```python
from build123d import *

# Parameters (mm, degrees)
BOSS_EXTRUDE1_OUTLINE_W   = 188.4
BOSS_EXTRUDE1_OUTLINE_H   = 88.4
BOSS_EXTRUDE1_DEPTH       = 5.8
BOSS_EXTRUDE1_2_OUTLINE_R = 1.5
BOSS_EXTRUDE1_2_OUTLINE_W = 22.55
BOSS_EXTRUDE1_2_OUTLINE_H = 11.95
BOSS_EXTRUDE1_2_DEPTH     = 5.8
SKETCH2_W                 = 22.55
SKETCH2_H                 = 11.95
CUT_EXTRUDE1_DEPTH        = 6.35
SKETCH3_R                 = 1.5
SKETCH3_W                 = 22.55
SKETCH3_H                 = 11.95
CUT_EXTRUDE2_DEPTH        = 107.804868803
CUT_EXTRUDE3_DEPTH        = 107.804868803
SKETCH5_W                 = 5.8
SKETCH5_H                 = 188.4
BOSS_EXTRUDE2_DEPTH       = 5.8
CUT_EXTRUDE5_DEPTH        = 5.8


# Read off the part's stored shape, not the designer's step: Boss-Extrude1
with BuildPart() as part:
    # Boss-Extrude1 outline → Boss-Extrude1 (new body)
    with BuildSketch(Plane(origin=(0, 0, 0), x_dir=(0, 0, -1), z_dir=(1, 0, 0))):
        Rectangle(BOSS_EXTRUDE1_OUTLINE_W, BOSS_EXTRUDE1_OUTLINE_H)
    extrude(amount=BOSS_EXTRUDE1_DEPTH)

    # Sketch2 → Cut-Extrude1 (cut)
    with BuildSketch(Plane(origin=(5.8, 0, 0), x_dir=(0, 0, -1), z_dir=(1, 0, 0))):
        with Locations((-70.783988916, 0)):
            Rectangle(SKETCH2_W, SKETCH2_H)
    extrude(amount=-CUT_EXTRUDE1_DEPTH, mode=Mode.SUBTRACT)

    # Sketch3 → Cut-Extrude2 (cut, through all)
    with BuildSketch(Plane(origin=(5.8, 0, 0), x_dir=(0, 0, -1), z_dir=(1, 0, 0))):
        with Locations((-66.978988916, 11)):
            Circle(SKETCH3_R)
        with Locations(Location((-66.978988916, -11, 0), (0, 0, 180))):
            Circle(SKETCH3_R)
        with Locations((-70.783988916, 0)):
            Rectangle(SKETCH3_W, SKETCH3_H)
    extrude(amount=-CUT_EXTRUDE2_DEPTH, mode=Mode.SUBTRACT)

    # Sketch4 → Cut-Extrude3 (cut, through all)
    with BuildSketch(Plane(origin=(5.8, 0, 0), x_dir=(0, 0, -1), z_dir=(1, 0, 0))):
        Polygon((-94.2, 34), (-90.2, 34), (-90.2, 35.21), (-87.85, 35.21), (-87.85, 34), (-85.85, 34), (-85.85, 31), (-87.85, 31), (-87.85, 29.79), (-90.2, 29.79), (-90.2, 31), (-94.2, 31), align=None)
        Polygon((-87.85, -31), (-87.85, -29.79), (-90.2, -29.79), (-90.2, -31), (-94.2, -31), (-94.2, -34), (-90.2, -34), (-90.2, -35.21), (-87.85, -35.21), (-87.85, -34), (-85.85, -34), (-85.85, -31), align=None)
        Polygon((94.2, -34), (90.2, -34), (90.2, -35.21), (87.85, -35.21), (87.85, -34), (85.85, -34), (85.85, -31), (87.85, -31), (87.85, -29.79), (90.2, -29.79), (90.2, -31), (94.2, -31), align=None)
        Polygon((87.85, 31), (87.85, 29.79), (90.2, 29.79), (90.2, 31), (94.2, 31), (94.2, 34), (90.2, 34), (90.2, 35.21), (87.85, 35.21), (87.85, 34), (85.85, 34), (85.85, 31), align=None)
    extrude(amount=-CUT_EXTRUDE3_DEPTH, mode=Mode.SUBTRACT)



with BuildPart() as body_2:
    # Boss-Extrude1 2 outline → Boss-Extrude1 2 (new body)
    with BuildSketch(Plane(origin=(0, 0, 0), x_dir=(0, 0, -1), z_dir=(1, 0, 0))):
        Polygon((94.2, 34), (94.2, 50), (-94.2, 50), (-94.2, 34), (-90.2, 34), (-90.2, 35.21), (-87.85, 35.21), (-87.85, 34), (-85.85, 34), (-85.85, 31), (-87.85, 31), (-87.85, 29.79), (-90.2, 29.79), (-90.2, 31), (-94.2, 31), (-94.2, -31), (-90.2, -31), (-90.2, -29.79), (-87.85, -29.79), (-87.85, -31), (-85.85, -31), (-85.85, -34), (-87.85, -34), (-87.85, -35.21), (-90.2, -35.21), (-90.2, -34), (-94.2, -34), (-94.2, -44.2), (94.2, -44.2), (94.2, -34), (90.2, -34), (90.2, -35.21), (87.85, -35.21), (87.85, -34), (85.85, -34), (85.85, -31), (87.85, -31), (87.85, -29.79), (90.2, -29.79), (90.2, -31), (94.2, -31), (94.2, 31), (90.2, 31), (90.2, 29.79), (87.85, 29.79), (87.85, 31), (85.85, 31), (85.85, 34), (87.85, 34), (87.85, 35.21), (90.2, 35.21), (90.2, 34), align=None)
        with Locations((-66.978988916, -11)):
            Circle(BOSS_EXTRUDE1_2_OUTLINE_R, mode=Mode.SUBTRACT)
        with Locations((-70.783988916, 0)):
            Rectangle(BOSS_EXTRUDE1_2_OUTLINE_W, BOSS_EXTRUDE1_2_OUTLINE_H, mode=Mode.SUBTRACT)
        with Locations((-66.978988916, 11)):
            Circle(BOSS_EXTRUDE1_2_OUTLINE_R, mode=Mode.SUBTRACT)
    extrude(amount=BOSS_EXTRUDE1_2_DEPTH)


with BuildPart() as part_1:
    add(part.part)

    add(body_2.part)  # Boss-Extrude2 merges body 2
    # Sketch5 → Boss-Extrude2 (add)
    with BuildSketch(Plane(origin=(0, 44.2, 0), x_dir=(1, 0, 0), z_dir=(0, 1, 0))):
        with Locations((2.9, 0)):
            Rectangle(SKETCH5_W, SKETCH5_H)
    extrude(amount=BOSS_EXTRUDE2_DEPTH)

    # Sketch8 → Cut-Extrude5 (cut)
    with BuildSketch(Plane(origin=(5.8, 0, 0), x_dir=(0, 0, -1), z_dir=(1, 0, 0))):
        with BuildLine():
            Line((-59.508988916, 4.5), (-59.508988916, -4.5))
            add(Edge.make_bspline(
                [(-59.508988916, -4.5), (-56.508988916, -4.5), (-56.508988916, 0), (-56.508988916, 4.5), (-59.508988916, 4.5)],
                knots=[3.141592654, 3.141592654, 3.141592654, 4.71238898, 4.71238898, 6.283185307, 6.283185307, 6.283185307], degree=2, weights=[1, 0.707106781, 1, 0.707106781, 1]))
        make_face()
    extrude(amount=-CUT_EXTRUDE5_DEPTH, mode=Mode.SUBTRACT)


solid = part_1.part
```
Geometry: final body of the model. Coordinates: model frame, mm. A direction names the side the tool comes from. Coordinates: 2 decimals unless noted, no trailing zeros.
Item 1: Material intervals for line 1 along Y through (x, z) = (2.4, 86.5); line 2 along Z through (x, y) = (2.4, -11); line 3 along Y through (x, z) = (2.9, 78) (3 decimals), sorted ascending.
Answer:
line 1: y = -44.2 to -34, -31 to 31, 34 to 50
line 2: z = -94.2 to 65.48, 68.48 to 94.2
line 3: y = -44.2 to -5.975, 5.975 to 50
Item 2: Access query for faces 1 (the face through (3, -34, -92)), 2 (the face through (3, -34, 92)), 3 (the face through (3, 5.975, 71)). Directions: +Z, -Z, +X, -X, +Y, -Y. A direction counts if a zero-diameter tool reaches every point of the face in a straight line with its end or side. Return the directions, or none.
Answer:
face 1: -Z, +X, -X
face 2: +Z, +X, -X
face 3: +X, -X
Item 3: Draft query along Z for faces 4 (the face through (3, -39, -94.2)), 5 (the face through (3, 34, -92)), 6 (the face through (3, -5.975, 71)). Return one class per face: released by +Z, released by -Z, zero draft, split by the parting line, or undercut.
Answer:
face 4: released by -Z
face 5: zero draft
face 6: undercut
Item 4: Section query A-A (x = 2.55). State how many separate pieces and enclosed holes the cut face has, then the cut area to 3 significant figures.
Answer:
separate pieces: 1
enclosed holes: 3
area: 17,300 mm2
